CAD build for the part. Positions are in the model's coordinates, mm. A direction names the side the tool comes from. Coordinates: 2 decimals unless noted, no trailing zeros. Write each loop counter-clockwise with the first axis right and the second up, starting at its lowest first coordinate (ties: lowest second). Pieces come first, ordered by that corner, then holes. Notation, with made-up numbers: (57, -24.5) - (87, -24.5) arc R9 ccw to (87, -17.5) - close; hole circle Ø5 at (-29, -18). An arc over 180 degrees is marked (long way). Answer in a Markdown table with one row per item. Add a question column.
Q1. Band-saw the part on A-A (x = 19). List the corners of the cut face in (y, z), and give its area (3 significant figures).
Q2. 3-axis set-ups, long thin cutter, end or side, ignore diameter. For faces 4 (the flat face through (30, 6, 0)), 5 (the cylindrical face through (9.577, 66.095, 0.867)): which of +Z, -Z, +X, -X, +Y, -Y reach the whole face in a straight line?
Q3. Drill centre lines: line 1 along Y through (x, z) = (14, 56); line 2 along X through (y, z) = (112, -45.5); line 3 along X through (y, z) = (16, -40). Where is each one in solid material? Low to high. Write a range as from..to.
Q4. Two-plate mould, pull along Z, no slides. Class faces 1 (the flat face through (4, 21, -46)), 2 (the cylindrical face through (1.97, -15.02, 47.69)), 3 (the flat face through (15, -4, -4)): +Z half, -Z half, draft (parallel to the pull), parting line (faces both ways), or undercut.
Q5. Pin check, flat tips, straight feed: pin 1 (2 mm diameter, centred on x = 33.5, y = 7.5, fed in from -Z); pin 2 (16 mm diameter, centred on y = 0, z = 0, fed in from +X); pin 3 (0.6 mm diameter, centred on x = 23.5, y = 7, fed in from +Z); pin 4 (13 mm diameter, centred on y = -4, z = -2, fed in from +X). Stop position of each tip, or through.
```python
from build123d import *

# Parameters (mm, degrees)
CUT_EXTRUDE_1_DEPTH      = 35
CUT_EXTRUDE_3_DEPTH      = 5
SKETCH_5_R               = 5
CUT_EXTRUDE_4_DEPTH      = 25
SKETCH_6_R               = 4
CUT_EXTRUDE_5_DEPTH      = 178.734491343
PATTERN_CIRCULAR_1_COUNT = 7
SKETCH_7_R               = 4
CUT_EXTRUDE_6_DEPTH      = 178.734491343
PATTERN_CIRCULAR_2_COUNT = 3


with BuildPart() as part:
    # Sketch 1 → Revolve 1 (revolve)
    with BuildSketch(Plane.XY, mode=Mode.PRIVATE) as revolve_1_sk:
        with BuildLine():
            Line((0, 0), (50, 0))
            Line((50, 0), (50, 12.5))
            Line((50, 12.5), (35, 12.5))
            ThreePointArc((35, 12.5), (20.857864376, 18.357864376), (15, 32.5))
            Line((15, 32.5), (15, 123.216373532))
            ThreePointArc((15, 123.216373532), (6.889116577, 112.845232579), (4, 100))
            Line((4, 100), (4, 50))
            Line((4, 50), (0, 50))
            Line((0, 50), (0, 0))
        make_face()
    revolve(revolve_1_sk.sketch.rotate(Axis((0, 0, 0), (1, 0, 0)), 90), axis=Axis((0, 0, 0), (1, 0, 0)))

    # Sketch 3 → Cut-Extrude 1 (cut)
    with BuildSketch(Plane(origin=(50, 0, 0), x_dir=(0, 0, -1), z_dir=(1, 0, 0))):
        with BuildLine():
            Line((-3, 6), (-3, 7.95298686))
            ThreePointArc((-3, 7.95298686), (-4.834769901, -6.991065727), (8.5, 0))
            ThreePointArc((8.5, 0), (6.991065727, 4.834769901), (3, 7.95298686))
            Line((3, 7.95298686), (3, 6))
            Line((3, 6), (-3, 6))
        make_face()
    extrude(amount=-CUT_EXTRUDE_1_DEPTH, mode=Mode.SUBTRACT)

    # Sketch 3_4 → Cut-Extrude 3 (cut)
    with BuildSketch(Plane(origin=(50, 0, 0), x_dir=(0, 0, -1), z_dir=(1, 0, 0))):
        with BuildLine():
            ThreePointArc((0, 8.5), (-1.524731401, 8.362128566), (-3, 7.95298686))
            Line((-3, 7.95298686), (-3, 6))
            Line((-3, 6), (0, 6))
            Line((0, 6), (0, 8.5))
        make_face()
        with BuildLine():
            ThreePointArc((3, 7.95298686), (1.524731401, 8.362128566), (0, 8.5))
            Line((0, 8.5), (0, 6))
            Line((0, 6), (3, 6))
            Line((3, 6), (3, 7.95298686))
        make_face()
    extrude(amount=-CUT_EXTRUDE_3_DEPTH, mode=Mode.SUBTRACT)

    # Sketch 5 → Cut-Extrude 4 (cut)
    with BuildSketch(Plane.ZY):
        Circle(SKETCH_5_R)
    extrude(amount=-CUT_EXTRUDE_4_DEPTH, mode=Mode.SUBTRACT)

    # Sketch 6 → Cut-Extrude 5 (cut, symmetric)
    with BuildSketch(Plane(origin=(15, 0, 0), x_dir=(0, 0, -1), z_dir=(1, 0, 0))):
        with Locations((0, 70)):
            Circle(SKETCH_6_R)
    cut_extrude_5 = extrude(amount=CUT_EXTRUDE_5_DEPTH, both=True, mode=Mode.SUBTRACT)

    # Pattern Circular 1: Cut-Extrude 5 ×7 about axis
    pattern_circular_1_axis = Axis((0, 0, 0), (1, 0, 0))
    for i in range(1, PATTERN_CIRCULAR_1_COUNT):
        add(cut_extrude_5.rotate(pattern_circular_1_axis, i * 360 / PATTERN_CIRCULAR_1_COUNT), mode=Mode.SUBTRACT)

    # Sketch 7 → Cut-Extrude 6 (cut, symmetric)
    with BuildSketch(Plane(origin=(15, 0, 0), x_dir=(0, 0, -1), z_dir=(1, 0, 0))):
        with Locations((0, 40)):
            Circle(SKETCH_7_R)
    cut_extrude_6 = extrude(amount=CUT_EXTRUDE_6_DEPTH, both=True, mode=Mode.SUBTRACT)

    # Pattern Circular 2: Cut-Extrude 6 ×3 about axis
    pattern_circular_2_axis = Axis((0, 0, 0), (1, 0, 0))
    for i in range(1, PATTERN_CIRCULAR_2_COUNT):
        add(cut_extrude_6.rotate(pattern_circular_2_axis, i * 360 / PATTERN_CIRCULAR_2_COUNT), mode=Mode.SUBTRACT)


solid = part.part
```
Checked values:
| question | item | result |
|---|---|---|
| 1 | outline | circle Ø41 at (0, 0); hole (6, -3) - (6, 3) - (7.95, 3) arc R8.5 ccw (long way) to (7.95, -3) - close |
| 1 | area | 1,110 mm² |
| 2 | face 4 | +X |
| 2 | face 5 | +X, -X |
| 3 | line 1 | y = -108.79..39.85, 47.44..108.79 |
| 3 | line 2 | x = 12.47..15 |
| 3 | line 3 | x = 0..15 |
| 4 | face 1 | draft |
| 4 | face 2 | parting line |
| 4 | face 3 | undercut |
| 5 | pin 1 | stops at z = -10.75 |
| 5 | pin 2 | stops at x = 45 |
| 5 | pin 3 | stops at z = 14.82 |
| 5 | pin 4 | stops at x = 50 |
